Part model, mm, in its own coordinate system. Face numbers are marked on the shaded views. A direction names the side the tool comes from. Give positions to 0.01 mm unless a question says otherwise; leave off trailing zeros. Order: outer loops, then holes, each group sorted by start corner. A loop starts at its lowest first (then second) coordinate and runs counter-clockwise, first axis right, second up. Notation, with made-up numbers: (-28.75, -17.75) - (26.25, -17.75) arc R30 ccw to (26.25, 21.25) - close; hole circle Ø8 at (57, 73.5). An arc over 180 degrees is marked (long way). Use one line per item in the form item = value. Start each with the question number.
1. Band-saw the part on C-C, the plane x = 2901. List the corners of the cut face in (y, z).
2. Band-saw the part on B-B, the plane y = 1604.5. List the corners of the cut face in (x, z).
3. Pin check, flat tip, straight feed: P1, Ø1.5, axis at x = 2907.5, y = 1607.5, coming from the +Z side. Stop position of the tip, or through.
4. Drill centre lines: line 1 (X direction, y = 1608.5, z = 4); line 2 (Y direction, x = 2891.5, z = 9.5); line 3 (Z direction, x = 2895, y = 1604.5). Where is each one in solid material? Low to high.
5. Pull direction X, two halves, no side cores. Call the marked faces 4, 5 and 6: +X half, -X half, draft (parallel to the pull), parting line (faces both ways), or undercut.
6. Band-saw the part on D-D, the plane z = -1. List the corners of the cut face in (x, y).
7. Tool access for the marked faces 1, 2 and 3: list every direction of +Z, -Z, +X, -X, +Y, -Y with a clear straight run to the whole face (end or side of a thin tool).
8. Band-saw the part on A-A, the plane z = 7. List the corners of the cut face in (x, y), plus the area to 3 significant figures.
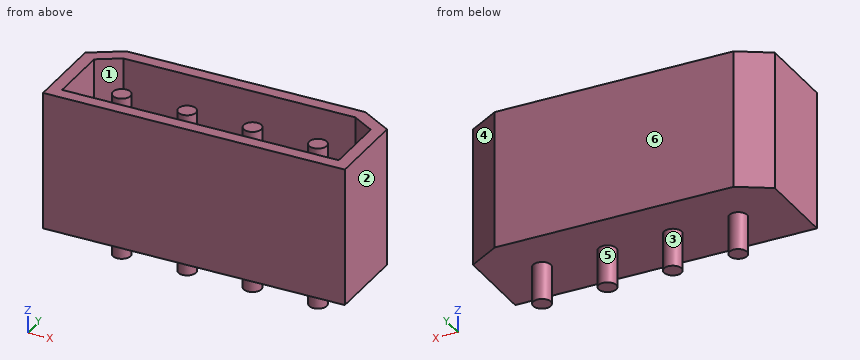
from build123d import *

# Parameters (mm, degrees)
EXTRUDE_1_DEPTH        = 11
CUT_EXTRUDE_1_DEPTH    = 9
SKETCH_3_R             = 0.7
EXTRUDE_2_DEPTH        = 8
SKETCH_4_R             = 1.576566923
CUT_EXTRUDE_2_DEPTH    = 3
PATTERN_LINEAR_1_COUNT = 4
PATTERN_LINEAR_1_PITCH = 5.2


with BuildPart() as part:
    # Model → 凸台-拉伸1 (new body)
    with BuildSketch(Plane.XY):
        Polygon((2890.278305735, 1611.212566626), (2909.278305735, 1611.212566626), (2911.778305735, 1609.712566626), (2911.778305735, 1603.212566626), (2887.778305735, 1603.212566626), (2887.778305735, 1609.712566626), align=None)
    extrude(amount=EXTRUDE_1_DEPTH)

    # 草图2 → 切除-拉伸1 (cut)
    with BuildSketch(Plane.XY.offset(11)):
        Polygon((2890.5552897, 1610.212566626), (2888.778305735, 1609.146376247), (2888.778305735, 1604.212566626), (2910.778305735, 1604.212566626), (2910.778305735, 1609.146376247), (2909.00132177, 1610.212566626), align=None)
    extrude(amount=-CUT_EXTRUDE_1_DEPTH, mode=Mode.SUBTRACT)

    # 草图3 → 凸台-拉伸2 (add, symmetric)
    with BuildSketch(Plane.XY.offset(2)):
        with Locations((2891.978305735, 1607.212566626)):
            Circle(SKETCH_3_R)
    extrude_2 = extrude(amount=EXTRUDE_2_DEPTH, both=True)

    # 草图4 → 切除-拉伸2 (cut)
    with BuildSketch(Plane(origin=(0, 0, -6), x_dir=(-1, 0, 0), z_dir=(0, 0, -1))):
        with Locations((-2891.978305735, 1607.212566626)):
            Circle(SKETCH_4_R)
    cut_extrude_2 = extrude(amount=-CUT_EXTRUDE_2_DEPTH, mode=Mode.SUBTRACT)

    # 阵列(线性)1: 凸台-拉伸2, 切除-拉伸2 ×4
    with Locations(*[(i * PATTERN_LINEAR_1_PITCH, 0, 0) for i in range(1, PATTERN_LINEAR_1_COUNT)]):
        add(extrude_2)
        add(cut_extrude_2, mode=Mode.SUBTRACT)


solid = part.part
From the geometry:
q1.outline = (1603.21, 0) - (1611.21, 0) - (1611.21, 11) - (1610.21, 11) - (1610.21, 2) - (1604.21, 2) - (1604.21, 11) - (1603.21, 11) - close
q2.outline = (2887.78, 0) - (2911.78, 0) - (2911.78, 11) - (2910.78, 11) - (2910.78, 2) - (2888.78, 2) - (2888.78, 11) - (2887.78, 11) - close
q3.P1 = 10
q4.line_1 = 2887.78 to 2888.78, 2910.78 to 2911.78
q4.line_2 = 1603.21 to 1604.21, 1606.7 to 1607.72, 1610.21 to 1611.21
q4.line_3 = 0 to 2
q5.face_4 = +X half
q5.face_5 = undercut
q5.face_6 = draft
q6.outline = circle Ø1.4 at (2891.98, 1607.21); circle Ø1.4 at (2897.18, 1607.21); circle Ø1.4 at (2902.38, 1607.21); circle Ø1.4 at (2907.58, 1607.21)
q7.face_1 = +Z
q7.face_2 = +Z, -Z, +X, +Y, -Y
q7.face_3 = -Z
q8.outline = (2887.78, 1603.21) - (2911.78, 1603.21) - (2911.78, 1609.71) - (2909.28, 1611.21) - (2890.28, 1611.21) - (2887.78, 1609.71) - close; circle Ø1.4 at (2891.98, 1607.21); circle Ø1.4 at (2897.18, 1607.21); circle Ø1.4 at (2902.38, 1607.21); circle Ø1.4 at (2907.58, 1607.21); hole (2888.78, 1604.21) - (2910.78, 1604.21) - (2910.78, 1609.15) - (2909, 1610.21) - (2890.56, 1610.21) - (2888.78, 1609.15) - close
q8.area = 64.3 mm²
